Could you check a few things on this drawing? It's one solid part, dimensions in mm from its lowest x, y, z. Give positions to 0.01 mm unless a question says otherwise; leave off trailing zeros. Write each loop counter-clockwise with the first axis right and the second up, starting at its lowest first coordinate (ties: lowest second). Pieces come first, ordered by that corner, then holes.
1. Suppose I cut it at D-D (y = 14). Please give me the cut outline in (x, z), and give its area (3 significant figures).
2. If I drill on probe 1 along Z at (x, y) = (10.25, 14) (1 decimal); probe 2 along Z at (x, y) = (8.5, 10.75) (1 decimal); probe 3 along X at (y, z) = (10.75, 16), over which ranges is the centre line in solid material (lowest first)?
3. I'm going to push flat-ended pins straight in: pin 1 (1 mm diameter, centred on y = 12, z = 13, fed in from -X) (1 decimal); pin 2 (5 mm diameter, centred on x = 20.5, y = 10, fed in from +Z); pin 3 (6 mm diameter, centred on x = 14, y = 3, fed in from +Z); pin 4 (12 mm diameter, centred on x = 16, z = 16.5, fed in from -Y). Where does each tip first touch, or does it pass through?
4. Thinking about a two-plate mould opening in Z: for the marked faces 1, 2 and 3, which applies, pulls with the +Z half, pulls with the -Z half, needs draft (parallel to the pull), parting line crosses it, or undercut?
5. Suppose I cut it at C-C (y = 6). Please give me the cut outline in (x, z).
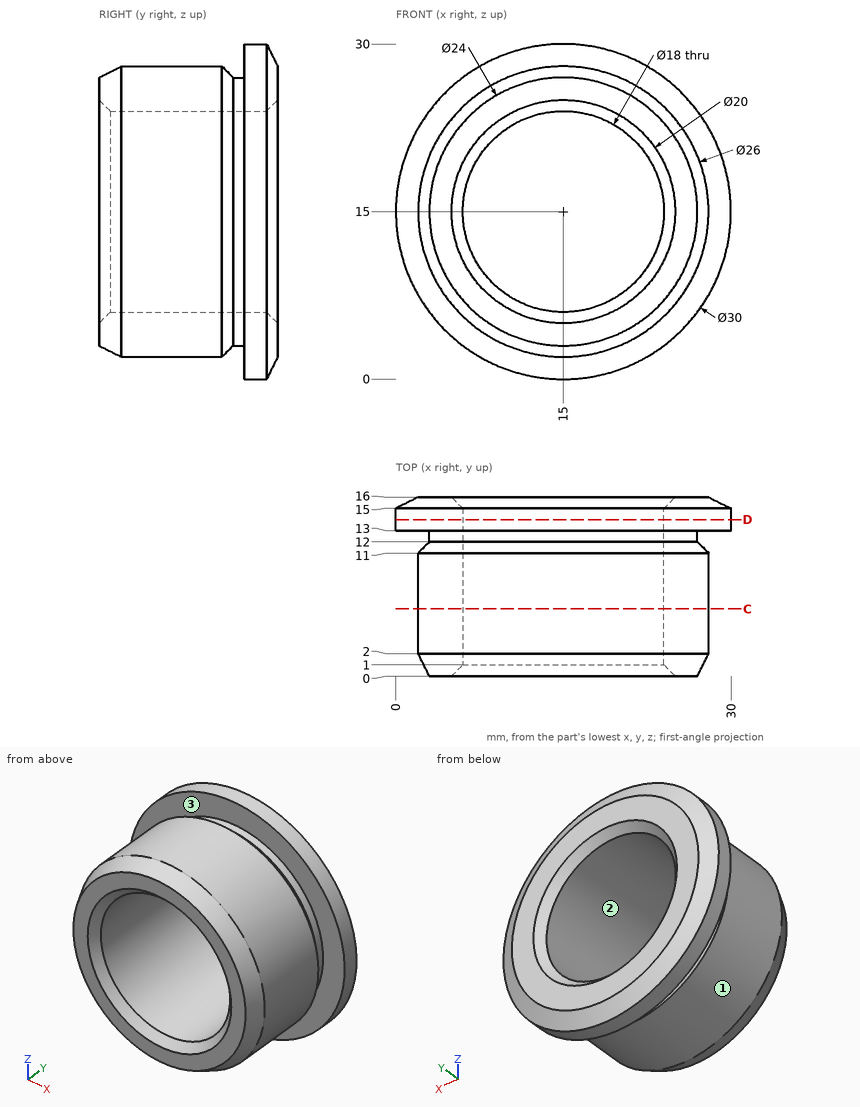
Checks:
1. outline: circle Ø30 at (15, 15); hole circle Ø18 at (15, 15)
1. area: 452 mm2
2. probe 1: z = 0.8 to 7.4, 22.6 to 29.2
2. probe 2: z = 3.7 to 8.8, 21.2 to 26.3
2. probe 3: x = 2.04 to 6.06, 23.94 to 27.96
3. pin 1: stops at x = 2.7
3. pin 2: stops at z = 27.65
3. pin 3: stops at z = 28
3. pin 4: passes through
4. face 1: parting line crosses it
4. face 2: undercut
4. face 3: needs draft
5. outline: circle Ø26 at (15, 15); hole circle Ø18 at (15, 15)
